For this review, take the finished solid that the model builds, in its own axes (mm). Coordinates: 2 decimals unless noted, no trailing zeros. Write each loop counter-clockwise with the first axis right and the second up, starting at its lowest first coordinate (ties: lowest second). Pieces come first, ordered by that corner, then holes. Notation, with made-up numbers: M -35,-29.5 L -20,-29.5 A32 cw -20,4.5 Z; hole C 17.25,86.25 d4. An arc over 180 degrees is marked long. Return JSON: item names as keys, results as strings.
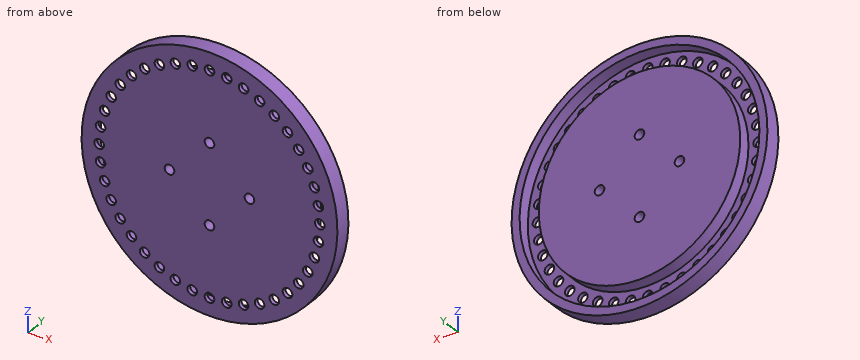
```python
from build123d import *

# Parameters (mm, degrees)
SKETCH1_R           = 40
SKETCH1_R_2         = 1.5
BOSS_EXTRUDE1_DEPTH = 5
SKETCH2_R           = 37.5
SKETCH2_R_2         = 31.5
CUT_EXTRUDE1_DEPTH  = 3.75


with BuildPart() as part:
    # Sketch1 → Boss-Extrude1 (new body)
    with BuildSketch(Plane(origin=(0, 0, 0), x_dir=(1, 0, 0), z_dir=(0, 1, 0))):
        with Locations(Location((0, 0, 0), (0, 0, 270))):
            Circle(SKETCH1_R)
        with Locations(Location((0, -34.5, 0), (0, 0, 270))):
            Circle(SKETCH1_R_2, mode=Mode.SUBTRACT)
        with Locations(Location((-5.396989044, -34.075247751, 0), (0, 0, 270))):
            Circle(SKETCH1_R_2, mode=Mode.SUBTRACT)
        with Locations(Location((-10.661086306, -32.811449812, 0), (0, 0, 270))):
            Circle(SKETCH1_R_2, mode=Mode.SUBTRACT)
        with Locations(Location((-15.662672241, -30.739725084, 0), (0, 0, 270))):
            Circle(SKETCH1_R_2, mode=Mode.SUBTRACT)
        with Locations(Location((-20.278591204, -27.911086306, 0), (0, 0, 270))):
            Circle(SKETCH1_R_2, mode=Mode.SUBTRACT)
        with Locations(Location((-24.395183951, -24.395183951, 0), (0, 0, 270))):
            Circle(SKETCH1_R_2, mode=Mode.SUBTRACT)
        with Locations(Location((-27.911086306, -20.278591204, 0), (0, 0, 270))):
            Circle(SKETCH1_R_2, mode=Mode.SUBTRACT)
        with Locations(Location((-30.739725084, -15.662672241, 0), (0, 0, 270))):
            Circle(SKETCH1_R_2, mode=Mode.SUBTRACT)
        with Locations(Location((-32.811449812, -10.661086306, 0), (0, 0, 270))):
            Circle(SKETCH1_R_2, mode=Mode.SUBTRACT)
        with Locations(Location((-34.075247751, -5.396989044, 0), (0, 0, 270))):
            Circle(SKETCH1_R_2, mode=Mode.SUBTRACT)
        with Locations(Location((-34.5, 0, 0), (0, 0, 270))):
            Circle(SKETCH1_R_2, mode=Mode.SUBTRACT)
        with Locations(Location((-34.075247751, 5.396989044, 0), (0, 0, 270))):
            Circle(SKETCH1_R_2, mode=Mode.SUBTRACT)
        with Locations(Location((-32.811449812, 10.661086306, 0), (0, 0, 270))):
            Circle(SKETCH1_R_2, mode=Mode.SUBTRACT)
        with Locations(Location((-30.739725084, 15.662672241, 0), (0, 0, 270))):
            Circle(SKETCH1_R_2, mode=Mode.SUBTRACT)
        with Locations(Location((-27.911086306, 20.278591204, 0), (0, 0, 270))):
            Circle(SKETCH1_R_2, mode=Mode.SUBTRACT)
        with Locations(Location((-24.395183951, 24.395183951, 0), (0, 0, 270))):
            Circle(SKETCH1_R_2, mode=Mode.SUBTRACT)
        with Locations(Location((-20.278591204, 27.911086306, 0), (0, 0, 270))):
            Circle(SKETCH1_R_2, mode=Mode.SUBTRACT)
        with Locations(Location((-15.662672241, 30.739725084, 0), (0, 0, 270))):
            Circle(SKETCH1_R_2, mode=Mode.SUBTRACT)
        with Locations(Location((-10.661086306, 32.811449812, 0), (0, 0, 270))):
            Circle(SKETCH1_R_2, mode=Mode.SUBTRACT)
        with Locations(Location((-5.396989044, 34.075247751, 0), (0, 0, 270))):
            Circle(SKETCH1_R_2, mode=Mode.SUBTRACT)
        with Locations(Location((0, 34.5, 0), (0, 0, 270))):
            Circle(SKETCH1_R_2, mode=Mode.SUBTRACT)
        with Locations(Location((5.396989044, 34.075247751, 0), (0, 0, 270))):
            Circle(SKETCH1_R_2, mode=Mode.SUBTRACT)
        with Locations(Location((10.661086306, 32.811449812, 0), (0, 0, 270))):
            Circle(SKETCH1_R_2, mode=Mode.SUBTRACT)
        with Locations(Location((15.662672241, 30.739725084, 0), (0, 0, 270))):
            Circle(SKETCH1_R_2, mode=Mode.SUBTRACT)
        with Locations(Location((20.278591204, 27.911086306, 0), (0, 0, 270))):
            Circle(SKETCH1_R_2, mode=Mode.SUBTRACT)
        with Locations(Location((24.395183951, 24.395183951, 0), (0, 0, 270))):
            Circle(SKETCH1_R_2, mode=Mode.SUBTRACT)
        with Locations(Location((27.911086306, 20.278591204, 0), (0, 0, 270))):
            Circle(SKETCH1_R_2, mode=Mode.SUBTRACT)
        with Locations(Location((30.739725084, 15.662672241, 0), (0, 0, 270))):
            Circle(SKETCH1_R_2, mode=Mode.SUBTRACT)
        with Locations(Location((32.811449812, 10.661086306, 0), (0, 0, 270))):
            Circle(SKETCH1_R_2, mode=Mode.SUBTRACT)
        with Locations(Location((34.075247751, 5.396989044, 0), (0, 0, 270))):
            Circle(SKETCH1_R_2, mode=Mode.SUBTRACT)
        with Locations(Location((34.5, 0, 0), (0, 0, 270))):
            Circle(SKETCH1_R_2, mode=Mode.SUBTRACT)
        with Locations(Location((34.075247751, -5.396989044, 0), (0, 0, 270))):
            Circle(SKETCH1_R_2, mode=Mode.SUBTRACT)
        with Locations(Location((32.811449812, -10.661086306, 0), (0, 0, 270))):
            Circle(SKETCH1_R_2, mode=Mode.SUBTRACT)
        with Locations(Location((30.739725084, -15.662672241, 0), (0, 0, 270))):
            Circle(SKETCH1_R_2, mode=Mode.SUBTRACT)
        with Locations(Location((27.911086306, -20.278591204, 0), (0, 0, 270))):
            Circle(SKETCH1_R_2, mode=Mode.SUBTRACT)
        with Locations(Location((24.395183951, -24.395183951, 0), (0, 0, 270))):
            Circle(SKETCH1_R_2, mode=Mode.SUBTRACT)
        with Locations(Location((20.278591204, -27.911086306, 0), (0, 0, 270))):
            Circle(SKETCH1_R_2, mode=Mode.SUBTRACT)
        with Locations(Location((15.662672241, -30.739725084, 0), (0, 0, 270))):
            Circle(SKETCH1_R_2, mode=Mode.SUBTRACT)
        with Locations(Location((10.661086306, -32.811449812, 0), (0, 0, 270))):
            Circle(SKETCH1_R_2, mode=Mode.SUBTRACT)
        with Locations(Location((5.396989044, -34.075247751, 0), (0, 0, 270))):
            Circle(SKETCH1_R_2, mode=Mode.SUBTRACT)
        with Locations(Location((0, -12.5, 0), (0, 0, 270))):
            Circle(SKETCH1_R_2, mode=Mode.SUBTRACT)
        with Locations(Location((-12.5, 0, 0), (0, 0, 270))):
            Circle(SKETCH1_R_2, mode=Mode.SUBTRACT)
        with Locations(Location((0, 12.5, 0), (0, 0, 270))):
            Circle(SKETCH1_R_2, mode=Mode.SUBTRACT)
        with Locations(Location((12.5, 0, 0), (0, 0, 270))):
            Circle(SKETCH1_R_2, mode=Mode.SUBTRACT)
    extrude(amount=BOSS_EXTRUDE1_DEPTH)

    # Sketch2 → Cut-Extrude1 (cut)
    with BuildSketch(Plane(origin=(0, 5, 0), x_dir=(1, 0, 0), z_dir=(0, 1, 0))):
        with Locations(Location((0, 0, 0), (0, 0, 270))):
            Circle(SKETCH2_R)
        with Locations(Location((0, 0, 0), (0, 0, 270))):
            Circle(SKETCH2_R_2, mode=Mode.SUBTRACT)
    extrude(amount=-CUT_EXTRUDE1_DEPTH, mode=Mode.SUBTRACT)


solid = part.part
```
1. Wall thickness on L1, parallel to Z at x = -10, y = 4; L2, parallel to Z at x = 14.5, y = 4.35; L3, parallel to X at y = 1.05, z = 30: over which ranges is each line inside the solid? List them lowest first. Write a range as from..to.
Checks:
{"L1": "-38.73..-36.14, -29.87..29.87, 36.14..38.73", "L2": "-37.28..-34.58, -27.96..27.96, 34.58..37.28", "L3": "-26.46..-16.97, -14.36..14.36, 16.97..26.46"}
2. We need section A-A (y = 4). State the section outline as (x, z) points.
Checks:
{"outline": "C 0,0 d80; C 0,0 d63; hole C 0,0 d75; hole C -12.5,0 d3; hole C 0,-12.5 d3; hole C 0,12.5 d3; hole C 12.5,0 d3"}
3. Clearance check with flat-ended pins moving along their axes: pin 1 Ø2.5 at (x, z) = (30.74, -15.66) entering from +Y; pin 2 Ø1.5 at (x, y) = (-14, 4.5) entering from -Z; pin 3 Ø3 at (y, z) = (3.5, 18.5) entering from +X; pin 4 Ø5 at (x, z) = (-27.91, 20.28) entering from +Y. State where each tip first meets the part, or that it passes through.
Checks:
{"pin 1": "through", "pin 2": "z = -37.74", "pin 3": "x = 36.21", "pin 4": "y = 1.25"}
